Build history of the part. All positions in model axes, mm. A direction names the side the tool comes from. Give positions to 0.01 mm unless a question says otherwise; leave off trailing zeros. Loops run counter-clockwise (first coordinate to the right, second up) from the corner with the lowest first, then second, coordinate; pieces in that order, holes last. Notation, with made-up numbers: M 59.25,12 L 93.25,12 A14 ccw 93.25,18 Z; hole C 72.5,71.5 d2. An arc over 180 degrees is marked long. Answer as a JSON object with one key per item and string values. Group by question number.
1. Slice it at C-C (z = 2). List the corners of the cut face in (x, y), then the cut area to 3 significant figures.
2. Slice it at D-D (x = 17.5). List the corners of the cut face in (y, z).
3. 3-axis set-ups, long thin cutter, end or side, ignore diameter. For faces 5 (the face through (9.5, -56.51, 15.65)), 6 (the face through (6, -42, -24.967)), 7 (the face through (0, -9, -21)), 8 (the face through (12.7, -9, -21)): which of +Z, -Z, +X, -X, +Y, -Y reach the whole face in a straight line?
4. Drop flat-ended pins along their axis: pin 1 Ø25 at (y, z) = (-18, -13) entering from +X; pin 2 Ø12 at (y, z) = (13.5, -51.5) entering from +X; pin 3 Ø7.5 at (x, z) = (6.35, 15.24) entering from +Y; pin 4 Ø5.5 at (x, y) = (6.35, 0) entering from +Z. Give the stop position or say it passes through.
5. Slice it at B-B (z = -40). List the corners of the cut face in (x, y), then the cut area to 3 significant figures.
6. Slice it at A-A (y = -38). List the corners of the cut face in (x, z), then the cut area to 3 significant figures.
7. Drill centre lines: line 1 along Y through (x, z) = (6.35, -57); line 2 along Y through (x, z) = (5.25, -46.5); line 3 along Z through (x, y) = (4, -55). Where is each one in solid material? Low to high. Write a range as [from, to].
8. Mould opens along X. For faces 1 (the face through (3.32, 17.14, -57.37)), 2 (the face through (8.496, -56.512, -43.07)), 3 (the face through (-6.35, -52.1, -31.5)), 4 (the face through (6, -30, 31.882)) say: released by +X, released by -X, zero draft, split by the parting line, or undercut.
from build123d import *

# Parameters (mm, degrees)
SKETCH1_R                = 20
BOSS_EXTRUDE1_DEPTH      = 12.7
BOSS_EXTRUDE2_DEPTH      = 6.35
BOSS_EXTRUDE2_DEPTH_BACK = 19.05
SKETCH2_R                = 3.175
CUT_EXTRUDE1_DEPTH       = 89.231203407
SKETCH10_R               = 3.175
CUT_EXTRUDE6_DEPTH       = 8.128
SKETCH4_W                = 20.078494948
SKETCH4_H                = 48.78095735
SKETCH4_W_2              = 48.420880553
SKETCH4_H_2              = 19.195923741
CUT_EXTRUDE2_DEPTH       = 26.162
SKETCH5_R                = 3.175
CUT_EXTRUDE3_DEPTH       = 11.43
SKETCH6_R                = 3.175
CUT_EXTRUDE4_DEPTH       = 11.43


with BuildPart() as part:
    # Sketch1 → Boss-Extrude1 (new body)
    with BuildSketch(Plane(origin=(0, 0, 0), x_dir=(0, 0, -1), z_dir=(1, 0, 0))):
        with BuildLine():
            Line((0, 31.882172919), (31.882172919, 31.882172919))
            Line((31.882172919, 31.882172919), (60.87463474, 31.882172919))
            Line((60.87463474, 31.882172919), (60.87463474, -60.96))
            Line((60.87463474, -60.96), (-31.882172919, -60.96))
            Line((-31.882172919, -60.96), (-31.882172919, 0))
            ThreePointArc((-31.882172919, 0), (-22.54410067, 22.54410067), (0, 31.882172919))
        make_face()
        Circle(SKETCH1_R, mode=Mode.SUBTRACT)
    extrude(amount=BOSS_EXTRUDE1_DEPTH)

    # Sketch8 → Boss-Extrude2 (add, two sides: drawn at the far end of the back side and taken through both)
    with BuildSketch(Plane(origin=(12.7, 0, 0), x_dir=(0, 0, -1), z_dir=(1, 0, 0)).offset(-BOSS_EXTRUDE2_DEPTH_BACK)):
        Polygon((60.87463474, 31.882172919), (53.770648903, 31.882172919), (53.770648903, -51.937867719), (-31.882172919, -51.937867719), (-31.882172919, -60.96), (53.770648903, -60.96), (60.87463474, -60.96), align=None)
    extrude(amount=BOSS_EXTRUDE2_DEPTH + BOSS_EXTRUDE2_DEPTH_BACK)

    # Sketch2 → Cut-Extrude1 (cut, through all)
    with BuildSketch(Plane(origin=(0, 0, 0), x_dir=(1, 0, 0), z_dir=(0, 1, 0))):
        with Locations(Location((6.35, 0, 0), (0, 0, 90))):
            Circle(SKETCH2_R)
    extrude(amount=CUT_EXTRUDE1_DEPTH, mode=Mode.SUBTRACT)

    # Sketch10 → Cut-Extrude6 (cut)
    with BuildSketch(Plane.XY.offset(31.882172919)):
        with Locations((6.35, 0)):
            Circle(SKETCH10_R)
    extrude(amount=-CUT_EXTRUDE6_DEPTH, mode=Mode.SUBTRACT)

    # Sketch4 → Cut-Extrude2 (cut)
    with BuildSketch(Plane.ZY):
        with Locations((-43.731401429, -0.427222634)):
            Rectangle(SKETCH4_W, SKETCH4_H)
        with Locations((-0.75610861, -42.339905849)):
            Rectangle(SKETCH4_W_2, SKETCH4_H_2)
        with Locations((-43.731401429, -42.339905849)):
            Rectangle(SKETCH4_W, SKETCH4_H_2)
    extrude(amount=-CUT_EXTRUDE2_DEPTH, mode=Mode.SUBTRACT)

    # Sketch5 → Cut-Extrude3 (cut)
    with BuildSketch(Plane(origin=(0, 0, -60.87463474), x_dir=(-1, 0, 0), z_dir=(0, 0, -1))):
        with Locations((-6.35, 16.187024645)):
            Circle(SKETCH5_R)
        with Locations((-6.35, -44.788648077)):
            Circle(SKETCH5_R)
    extrude(amount=-CUT_EXTRUDE3_DEPTH, mode=Mode.SUBTRACT)

    # Sketch6 → Cut-Extrude4 (cut)
    with BuildSketch(Plane.XZ.offset(60.96)):
        with Locations(Location((6.35, 15.24, 0), (0, 0, 270))):
            Circle(SKETCH6_R)
        with Locations(Location((6.35, -45.41055385, 0), (0, 0, 270))):
            Circle(SKETCH6_R)
    extrude(amount=-CUT_EXTRUDE4_DEPTH, mode=Mode.SUBTRACT)


solid = part.part
Established:
{
 "1": {"outline": "M -6.35,-60.96 L 19.05,-60.96 L 19.05,-51.94 L -6.35,-51.94 Z; M 0,-32.74 L 12.7,-32.74 L 12.7,-19.9 L 0,-19.9 Z; M 0,19.9 L 3.88,19.9 L 3.88,31.82 L 0,31.82 Z; M 8.82,19.9 L 12.7,19.9 L 12.7,31.82 L 8.82,31.82 Z", "area": "485 mm^2"},
 "2": {"outline": "M -60.96,-60.87 L 31.88,-60.87 L 31.88,-53.77 L -51.94,-53.77 L -51.94,31.88 L -60.96,31.88 Z"},
 "3": {"face 5": "-Y", "face 6": "+X, -X", "face 7": "+Z, -X, +Y", "face 8": "+Z, +X, +Y"},
 "4": {"pin 1": "stops at x = 12.7", "pin 2": "stops at x = 19.05", "pin 3": "stops at y = 29.74", "pin 4": "stops at z = 23.75"},
 "5": {"outline": "M -6.35,-60.96 L 19.05,-60.96 L 19.05,-51.94 L -6.35,-51.94 Z; M 0,-32.74 L 12.7,-32.74 L 12.7,-24.82 L 0,-24.82 Z; M 0,23.96 L 12.7,23.96 L 12.7,31.88 L 0,31.88 Z", "area": "430 mm^2"},
 "6": {"outline": "M -6.35,-60.87 L 19.05,-60.87 L 19.05,-53.77 L -6.35,-53.77 Z; M 0,-33.69 L 12.7,-33.69 L 12.7,-24.97 L 0,-24.97 Z; M 0,23.45 L 12.7,23.45 L 12.7,31.88 L 0,31.88 Z", "area": "398 mm^2"},
 "7": {"line 1": "y = [-60.96, -47.96], [-41.61, 13.01], [19.36, 31.88]", "line 2": "y = [-32.74, -24.82], [23.96, 31.88]", "line 3": "z = [-60.87, -47.55], [-43.28, 13.11], [17.37, 31.88]"},
 "8": {"face 1": "undercut", "face 2": "undercut", "face 3": "released by -X", "face 4": "zero draft"}
}
